Input: part model. Units: mm. Frame: model coordinates. A direction names the side the tool comes from. Give positions to 0.01 mm unless a question says otherwise; leave off trailing zeros. Order: outer loops, then holes, each group sorted by start corner. A loop starts at its lowest first (then second) coordinate and runs counter-clockwise, first axis right, second up. Notation, with made-up numbers: (-6.75, 33.25) - (28.25, 33.25) arc R32 cw to (28.25, 66.25) - close; hole circle Ø8 at (45, -16). An arc over 180 degrees is marked (long way). Use a Markdown table: item, result.
Autodesk Inventor part; units mm, degrees
ref_plane "Work Plane1" through (29, 0, 0) normal (0, -1, 0) x (1, 0, 0)
ref_plane "YZ Plane" through (0, 0, 0) normal (1, 0, 0) x (0, 1, 0)
ref_plane "XZ Plane" through (0, 0, 0) normal (0, 1, 0) x (-1, 0, 0)
sketch "Sketch1" plane through (0, 0, 0) normal (0, 0, 1) x (1, 0, 0)
  line L0 (0.2879, 0) -> (25.4, 0)
  line L1 (25.4, 0) -> (25.4, 2.413)
  line L2 (25.4, 2.413) -> (2.1084, 2.413)
  line L3 (2.1084, 2.413) -> (0.0001, 2.413)
  line L4 (0.0001, 2.413) -> (0, 2.413)
  line L5 (0, 2.413) -> (0, 4.5847)
  line L6 (0, 4.5847) -> (-2.5654, 4.5847)
  line L7 (-2.5654, 4.5847) -> (-2.5654, 1.8624)
  line L8 (-2.5654, 1.8624) -> (-0.7874, 1.8624)
  line L9 (-0.7874, 1.8624) -> (0.2879, 0)
  line L10 (-8.1585, 0) -> (30.9931, 0)
  line L11 (0, -0.9169) -> (0, 5.5016)
  line L12 (2.1084, 2.413) -> (0, 2.413) construction
  dimension "d1" = 23.2916
  dimension "d2" = 2.1083
  dimension "d3" = 2.5654
  dimension "d4" = 1.778
  dimension "d5" = 60
  dimension "d6" = 4.826
  dimension "d7" = 4.826
  dimension "d8" = 3.7248
  dimension "d9" = 9.1694
  dimension "d26" = 25.4
revolve "Body" add sketch "Sketch1" angle 360 about axis through (0.2879, 0, 0) along (1, 0, 0) contours L9 L11 L3 L2 L1 L0 | L9 L8 L7 L6 L5 L11
sketch "Sketch2" plane through (-2.5654, 0, 0) normal (-1, 0, 0) x (0, 0, 1)
  circle A0 centre (0, 0) radius 1.8624
  line L0 (0, -6.4186) -> (0, 6.4186)
  line L1 (-6.4186, 0) -> (6.4186, 0)
  line L2 (1.8624, 0) -> (0.9312, -1.6129)
  line L3 (0.9312, -1.6129) -> (-0.9312, -1.6129)
  line L4 (-0.9312, -1.6129) -> (-1.8624, 0)
  line L5 (-1.8624, 0) -> (-0.9312, 1.6129)
  line L6 (-0.9312, 1.6129) -> (0.9312, 1.6129)
  line L7 (0.9312, 1.6129) -> (1.8624, 0)
extrude "Slot" add sketch "Sketch2" against normal up to next contours L7 A0 | A0 L2 | L6 L0 A0 | A0 L0 L3 | L0 L6 A0 | A0 L3 L0 | L4 A0 | A0 L5
fillet "Fillet1" radius 2.0574 1 edges at (-2.5654, -4.5847, 0)
thread "Thread"
chamfer "Chamfer1" distance 0.4724 distance2 0.4724 1 edges at (25.4, -2.413, 0) measured on face at (25.4, 0.9527, 0.2826)
ref_plane "Work Plane1" through (29, 0, 0) normal (0, -1, 0) x (1, 0, 0)
fillet "Fillet2" radius 0.1 1 edges at (0.0001, -2.413, 0)
equation "\"d30\" = R"
equation "\"d17\" = RR"
equation "\"d13\" = GEL"
equation "\"d15\" = -0.5 * SPD + 0.5 * GD"
equation "\"d16\" = GUL"
equation "\"d1\" = GEL"
equation "\"d3\" = KOH"
equation "\"d4\" = INTI"
equation "\"d6\" = GD"
equation "\"d7\" = BDM"
equation "\"d8\" = 1.1547 * SW"
equation "\"d9\" = KOD"
equation "\"d26\" = NLG"
equation "\"GD\" = NND"
equation "\"NLG\" = 25.4"
equation "\"GEL\" = 23.2916"
equation "\"KOD\" = 9.1694"
equation "\"KOH\" = 2.5654"
equation "\"INTI\" = 1.778"
equation "\"GAL\" = 2.1082"
equation "\"GUL\" = 0.47244"
equation "\"BDM\" = NND"
equation "\"SW\" = 3.2258"
equation "\"RR\" = 2.0574"
equation "\"SPD\" = 3.88112"
equation "\"R\" = 0.1"
equation "\"TOA\" = 30deg"
equation "\"GD1\" = SPD"
equation "\"THREADDIA\" = 4.826"
equation "\"KOH1\" = 0.508"
equation "\"NND\" = 4.826"
equation "\"E0\" = 3.72593"
properties part number "ANSI B18.3 - No. 10-32 - 1, HSBHCSI" material "Steel, Mild"
1. Material intervals for line 1 along X through (y, z) = (-0.75, -4); line 2 along Y through (x, z) = (10, 1); line 3 along X through (y, z) = (2.5, 1.5), sorted ascending.
Response:
| item | result |
|---|---|
| line 1 | x = -1.87 to 0 |
| line 2 | y = -2.2 to 2.2 |
| line 3 | x = -2.53 to 0 |
2. Mould query, pull axis Z, two halves, no side actions, for faces 1 (the face through (-1.6, 0.8, 1.4)), 2 (the face through (-0.26, -3.64, 2.79)), 3 (the face through (25.4, 0, 0)). Classes: pulls with the +Z half, pulls with the -Z half, needs draft (parallel to the pull), parting line crosses it, or undercut.
Response:
| item | result |
|---|---|
| face 1 | undercut |
| face 2 | parting line crosses it |
| face 3 | needs draft |
3. Set-up query: faces 4 (the face through (-2.565, -2, 0)), 5 (the face through (12.34, -1.915, 1.468)), 6 (the face through (-1.6, -0.8, 1.4)). Return all of +Z, -Z, +X, -X, +Y, -Y with unobstructed straight access to the full face (end or side cutting, diameter ignored); none if empty.
Response:
| item | result |
|---|---|
| face 4 | +Z, -Z, -X, +Y, -Y |
| face 5 | +X |
| face 6 | -X |
4. Section query A-A (x = 11.5). Return loops of the section in (y, z).
Response:
| item | result |
|---|---|
| outline | circle Ø4.83 at (0, 0) |
5. Pin query (flat end, axial travel): pin 1 (4 mm diameter, centred on x = 15.5, y = 1, fed in from -Z); pin 2 (3 mm diameter, centred on x = 20.5, z = 0.5, fed in from +Y); pin 3 (3 mm diameter, centred on x = 17, z = -3.5, fed in from -Y). Return the tip coordinate at first contact, or that it passes through.
Response:
| item | result |
|---|---|
| pin 1 | stops at z = -2.41 |
| pin 2 | stops at y = 2.41 |
| pin 3 | stops at y = -1.35 |
